Design review of the part built by this model. Coordinates are the model's own, in mm. Face numbers are marked on the shaded views. A direction names the side the tool comes from. Coordinates: 2 decimals unless noted, no trailing zeros. Loops run counter-clockwise (first coordinate to the right, second up) from the corner with the lowest first, then second, coordinate; pieces in that order, holes last. Notation, with made-up numbers: M 57.25,28.25 L 102.25,28.25 A23 ccw 102.25,67.25 Z; hole C 66.5,83 d8. An arc over 180 degrees is marked long. Put each result on its own line as item: value. Start each with the question number.
(1) For probe 1 along Z at (x, y) = (-12, -8.5); probe 2 along Y at (x, z) = (12.5, 7); probe 3 along Z at (x, y) = (20, -8), list the stretches that pass through material, from the lowest coordinate up. Write a range as [from, to].
(2) Take a section at C-C, the plane y = -13. Give the boundary of the cut face in (x, z).
(3) Take a section at A-A, the plane x = 0. Give the boundary of the cut face in (y, z).
(4) Take a section at B-B, the plane z = 2. Give the boundary of the cut face in (x, y), then the cut area to 3 significant figures.
(5) Take a section at D-D, the plane x = 18.5. Give the boundary of the cut face in (y, z).
(6) Clearance check with flat-ended pins moving along their axes: pin 1 (3 mm diameter, centred on x = -1, z = -17.5, fed in from +Y); pin 2 (10 mm diameter, centred on y = -8, z = -3.5, fed in from +X); pin 3 (11 mm diameter, centred on x = -3, z = 23, fed in from +Y); pin 4 (3 mm diameter, centred on x = 14, z = -2, fed in from +Y). State where each tip first meets the part, or that it passes through.
(7) For the marked faces 1, 2 and 3, list the 3-axis set-ups (+Z, -Z, +X, -X, +Y, -Y) from which the entire face can be reached by the end or side of a thin tool; tool diameter is ignored.
```python
from build123d import *

# Parameters (mm, degrees)
F1_DEPTH = 15
F3_DEPTH = 15
F4_R     = 7.5
F5_DEPTH = 25


with BuildPart() as f1:
    # F0 (on Top) → F1 (new body)
    with BuildSketch(Plane.XY):
        with BuildLine():
            ThreePointArc((22.5, 0), (17.960155, 10.960155), (7, 15.5))
            Line((7, 15.5), (-7, 15.5))
            ThreePointArc((-7, 15.5), (-17.960155, 10.960155), (-22.5, 0))
            Line((-22.5, 0), (-7, 0))
            Line((-7, 0), (0, 0))
            Line((0, 0), (7, 0))
            Line((7, 0), (22.5, 0))
        make_face()
        with BuildLine():
            ThreePointArc((7, -15.5), (17.960155, -10.960155), (22.5, 0))
            Line((22.5, 0), (7, 0))
            Line((7, 0), (0, 0))
            Line((0, 0), (-7, 0))
            Line((-7, 0), (-22.5, 0))
            ThreePointArc((-22.5, 0), (-17.960155, -10.960155), (-7, -15.5))
            Line((-7, -15.5), (7, -15.5))
        make_face()
    extrude(amount=F1_DEPTH)

    # F2 (on face) → F3 (join)
    with BuildSketch(Plane.XY.offset(15)):
        with BuildLine():
            ThreePointArc((21.5, 0), (17.253048, 10.253048), (7, 14.5))
            Line((7, 14.5), (-7, 14.5))
            ThreePointArc((-7, 14.5), (-17.253048, 10.253048), (-21.5, 0))
            Line((-21.5, 0), (-7, 0))
            Line((-7, 0), (0, 0))
            Line((0, 0), (7, 0))
            Line((7, 0), (21.5, 0))
        make_face()
        with BuildLine():
            ThreePointArc((7, -14.5), (17.253048, -10.253048), (21.5, 0))
            Line((21.5, 0), (7, 0))
            Line((7, 0), (0, 0))
            Line((0, 0), (-7, 0))
            Line((-7, 0), (-21.5, 0))
            ThreePointArc((-21.5, 0), (-17.253048, -10.253048), (-7, -14.5))
            Line((-7, -14.5), (7, -14.5))
        make_face()
    extrude(amount=F3_DEPTH)

    # F4 (on face) → F5 (join)
    with BuildSketch(Plane(origin=(0, 0, 0), x_dir=(1, 0, 0), z_dir=(0, 0, -1))):
        Circle(F4_R)
    extrude(amount=F5_DEPTH)


solid = f1.part
```
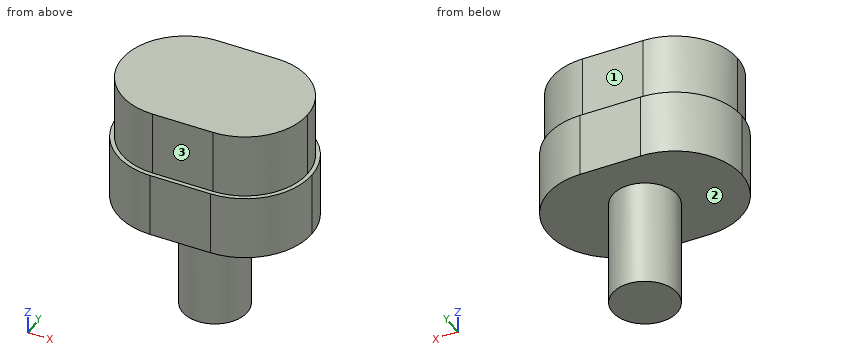
Computed values:
1. probe 1: z = [0, 30]
1. probe 2: y = [-14.49, 14.49]
1. probe 3: z = [0, 15]
2. outline: M -15.44,0 L 15.44,0 L 15.44,15 L 13.42,15 L 13.42,30 L -13.42,30 L -13.42,15 L -15.44,15 Z
3. outline: M -15.5,0 L -7.5,0 L -7.5,-25 L 7.5,-25 L 7.5,0 L 15.5,0 L 15.5,15 L 14.5,15 L 14.5,30 L -14.5,30 L -14.5,15 L -15.5,15 Z
4. outline: M -7,-15.5 L 7,-15.5 A15.5 ccw 7,15.5 L -7,15.5 A15.5 ccw Z
4. area: 1,190 mm^2
5. outline: M -10.39,0 L 10.39,0 L 10.39,15 L 8.83,15 L 8.83,30 L -8.83,30 L -8.83,15 L -10.39,15 Z
6. pin 1: stops at y = 7.5
6. pin 2: stops at x = 21.85
6. pin 3: stops at y = 14.5
6. pin 4: passes through
7. face 1: +Z, +X, -X, +Y
7. face 2: -Z
7. face 3: +Z, +X, -X, -Y
